```python
from build123d import *

# Parameters (mm, degrees)
SKETCH1_R           = 16
SKETCH1_R_2         = 2.5
BOSS_EXTRUDE1_DEPTH = 5
CHAMFER1_SIZE       = 2
FILLET1_R           = 0.5


with BuildPart() as part:
    # Sketch1 → Boss-Extrude1 (new body)
    with BuildSketch(Plane(origin=(0, 0, 0), x_dir=(1, 0, 0), z_dir=(0, 1, 0))):
        Circle(SKETCH1_R)
        Circle(SKETCH1_R_2, mode=Mode.SUBTRACT)
    extrude(amount=BOSS_EXTRUDE1_DEPTH)

    # Chamfer1
    chamfer1_edges = [part.edges().sort_by_distance(p)[0] for p in [
        (-2.5, 5, 0),
    ]]
    chamfer(chamfer1_edges, length=CHAMFER1_SIZE)

    # Fillet1
    fillet1_edges = [part.edges().sort_by_distance(p)[0] for p in [
        (-16, 0, 0),
        (-16, 5, 0),
    ]]
    fillet(fillet1_edges, radius=FILLET1_R)


solid = part.part
```
CAD build for the part. Positions are in the model's coordinates, mm. Round coordinates to 2 decimals unless told otherwise and drop trailing zeros. Write each loop counter-clockwise with the first axis right and the second up, starting at its lowest first coordinate (ties: lowest second). Pieces come first, ordered by that corner, then holes. Notation, with made-up numbers: (-16, 50) -> (33, 50) arc R19 ccw to (33, 86) -> close; hole circle Ø7 at (-16, 42.5). An arc over 180 degrees is marked (long way). Answer in a Markdown table with one row per item. Add a question column.
Item 1: Drill centre lines: line 1 (Z direction, x = 0, y = 2.1); line 2 (Z direction, x = -0.5, y = 2.4). Where is each one in solid material? Low to high. Write a range as from..to.
Item 2: Drop flat-ended pins along their axis: pin 1 Ø1.5 at (y, z) = (4, 1) entering from -X; pin 2 Ø2 at (y, z) = (3.5, 12.5) entering from -X; pin 3 Ø1 at (y, z) = (2.5, 7.5) entering from -X. Give the stop position or say it passes through.
Item 3: Mould opens along Z. For faces 1 (the face through (-0.54, 1.48, 2.44)), 2 (the face through (-0.569, 3.125, 2.563)), 3 (the face through (3, 0, 0)), 4 (the face through (-3.47, 2.47, 15.62)) say: pulls with the +Z half, pulls with the -Z half, needs draft (parallel to the pull), parting line crosses it, or undercut.
Item 4: Saw through at B-B, the plane z = 0. Write the cut outline in (x, y).
Item 5: Saw through at A-A, the plane x = 0. Write the cut outline in (y, z).
Findings below:
| question | item | result |
|---|---|---|
| 1 | line 1 | z = -16..-2.5, 2.5..16 |
| 1 | line 2 | z = -15.99..-2.45, 2.45..15.99 |
| 2 | pin 1 | stops at x = -16 |
| 2 | pin 2 | stops at x = -11.12 |
| 2 | pin 3 | stops at x = -14.39 |
| 3 | face 1 | undercut |
| 3 | face 2 | undercut |
| 3 | face 3 | needs draft |
| 3 | face 4 | parting line crosses it |
| 4 | outline | (-16, 0.5) arc R0.5 ccw to (-15.5, 0) -> (-2.5, 0) -> (-2.5, 3) -> (-4.5, 5) -> (-15.5, 5) arc R0.5 ccw to (-16, 4.5) -> close; (2.5, 0) -> (15.5, 0) arc R0.5 ccw to (16, 0.5) -> (16, 4.5) arc R0.5 ccw to (15.5, 5) -> (4.5, 5) -> (2.5, 3) -> close |
| 5 | outline | (0, -15.5) arc R0.5 ccw to (0.5, -16) -> (4.5, -16) arc R0.5 ccw to (5, -15.5) -> (5, -4.5) -> (3, -2.5) -> (0, -2.5) -> close; (0, 2.5) -> (3, 2.5) -> (5, 4.5) -> (5, 15.5) arc R0.5 ccw to (4.5, 16) -> (0.5, 16) arc R0.5 ccw to (0, 15.5) -> close |
